Part print with two shaded views. Sizes in mm from the minimum x, y, z corner. A direction names the side the tool comes from. Round coordinates to 2 decimals unless told otherwise and drop trailing zeros. Order: outer loops, then holes, each group sorted by start corner. A loop starts at its lowest first (then second) coordinate and runs counter-clockwise, first axis right, second up. Notation, with made-up numbers: M 32.25,16 L 61.25,16 A24 cw 61.25,34 Z; hole C -19,-5.75 d3. An arc over 180 degrees is marked long. One line per question, with ' | ' between items. Start each with the question number.
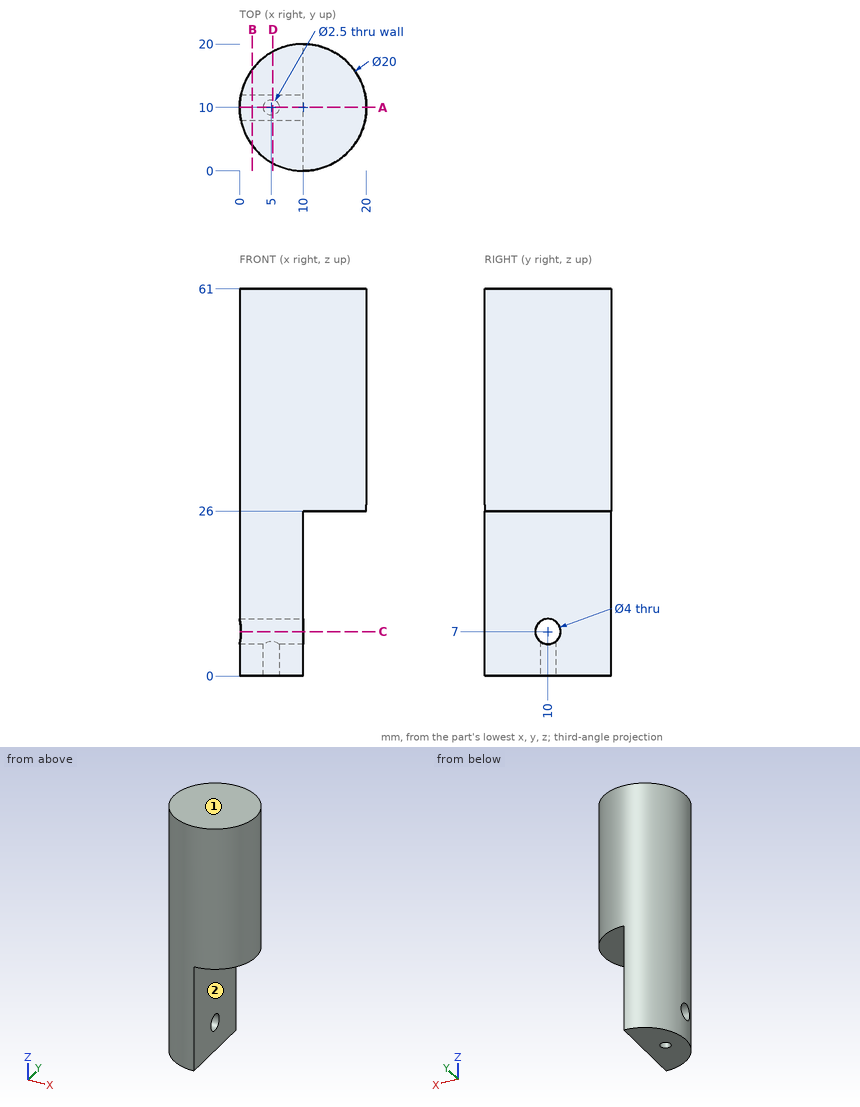
Item 1: Cut at C-C on z = 7. Write the cut outline in (x, y).
Item 2: Cut at A-A on y = 10. Write the cut outline in (x, z).
Item 3: Cut at B-B on x = 2. Write the cut outline in (y, z).
Item 4: Cut at D-D on x = 5.25. Write the cut outline in (y, z).
Item 5: Wall check: line 1 along Z through (x, y) = (16.75, 8); line 2 along Y through (x, z) = (2.5, 7); line 3 along Y through (x, z) = (2.75, 7). Give the ranges that are in metal, low to high. Write a range as [from, to].
Item 6: Tool access for the marked faces 1 and 2: list every direction of +Z, -Z, +X, -X, +Y, -Y with a clear straight run to the whole face (end or side of a thin tool).
Item 7: Flat gauge pins, fed straight in: pin 1 (5 mm diameter, centred on y = 10, z = 7, fed in from +X); pin 2 (1.5 mm diameter, centred on x = 3.5, z = 47.5, fed in from +Y); pin 3 (2 mm diameter, centred on x = 9.5, z = 39.5, fed in from -Y); pin 4 (8 mm diameter, centred on x = 15, y = 14, fed in from -Z). Where does each tip first touch, or does it go through?
Results found:
1) outline: M 0.2,8 A10 ccw 10,0 L 10,8 Z; M 0.2,12 L 10,12 L 10,20 A10 ccw Z
2) outline: M 0,0 L 3.75,0 L 3.75,5 L 0,5 Z; M 0,9 L 10,9 L 10,26 L 20,26 L 20,61 L 0,61 Z; M 6.25,0 L 10,0 L 10,5 L 6.25,5 Z
3) outline: M 4,0 L 16,0 L 16,61 L 4,61 Z; hole C 10,7 d4
4) outline: M 1.2,0 L 8.78,0 L 8.78,5.42 A2 cw long 11.22,5.42 L 11.22,0 L 18.8,0 L 18.8,61 L 1.2,61 Z
5) line 1: z = [26, 61] | line 2: y = [3.39, 8], [12, 16.61] | line 3: y = [3.11, 8], [12, 16.89]
6) face 1: +Z, +X, -X, +Y, -Y | face 2: -Z, +X, +Y, -Y
7) pin 1: stops at x = 10 | pin 2: stops at y = 18.18 | pin 3: stops at y = 0 | pin 4: stops at z = 26
